```python
from build123d import *

# Parameters (mm, degrees)
SKETCH_1_W          = 15
SKETCH_1_H          = 3
SKETCH_2_R          = 2.1
CUT_EXTRUDE_1_DEPTH = 10


with BuildPart() as part:
    # 草图1 → 旋转1 (revolve)
    with BuildSketch(Plane.XY, mode=Mode.PRIVATE) as revolve_1_sk:
        with Locations((83.58, 1.5)):
            Rectangle(SKETCH_1_W, SKETCH_1_H)
    revolve(revolve_1_sk.sketch.rotate(Axis((0, 0, 0), (0, 1, 0)), 90), axis=Axis((0, 0, 0), (0, 1, 0)))

    # 草图2 → 切除-拉伸1 (cut)
    with BuildSketch(Plane(origin=(0, 3, 0), x_dir=(1, 0, 0), z_dir=(0, 1, 0))):
        with Locations(Location((-83.9, 0, 0), (0, 0, 270))):
            Circle(SKETCH_2_R)
        with Locations(Location((-59.326258942, 59.326258942, 0), (0, 0, 270))):
            Circle(SKETCH_2_R)
        with Locations(Location((0, 83.9, 0), (0, 0, 270))):
            Circle(SKETCH_2_R)
        with Locations(Location((59.326258942, 59.326258942, 0), (0, 0, 270))):
            Circle(SKETCH_2_R)
        with Locations(Location((83.9, 0, 0), (0, 0, 270))):
            Circle(SKETCH_2_R)
        with Locations(Location((59.326258942, -59.326258942, 0), (0, 0, 270))):
            Circle(SKETCH_2_R)
        with Locations(Location((0, -83.9, 0), (0, 0, 270))):
            Circle(SKETCH_2_R)
        with Locations(Location((-59.326258942, -59.326258942, 0), (0, 0, 270))):
            Circle(SKETCH_2_R)
    extrude(amount=-CUT_EXTRUDE_1_DEPTH, mode=Mode.SUBTRACT)


solid = part.part
```
Geometry check sheet. Reference: the model listing, model coordinates, mm. Give positions to 0.01 mm unless a question says otherwise; leave off trailing zeros. Order: outer loops, then holes, each group sorted by start corner. A loop starts at its lowest first (then second) coordinate and runs counter-clockwise, first axis right, second up. Notation, with made-up numbers: (48, 61.25) - (95, 61.25) arc R12 ccw to (95, 66.25) - close; hole circle Ø2 at (67, 41). An arc over 180 degrees is marked (long way). Answer in a Markdown table with one row per item. Add a question column.
Q1. Mould release check, pull along Z, two halves, no side actions. Record for faces 1 (the cylindrical face through (-27.358, 1.521, -86.874)), 2 (the flat face through (-54, 0, 54)), 3 (the cylindrical face through (-60.604, 1.521, -60.993)): pulls with the +Z half, pulls with the -Z half, needs draft (parallel to the pull), parting line crosses it, or undercut.
Q2. Material ranges on probe 1 along X at (y, z) = (1, 0); probe 2 along Z at (x, y) = (-1.5, 2.55); probe 3 along X at (y, z) = (0.3, -1), recorded low to high. Write a range as from..to.
Q3. Cross-section at B-B, the plane z = -63.5. Enter the section's corners in (x, y).
Q4. Cross-section at A-A, the plane x = 52. Enter the section's corners in (y, z), then the cut area to 3 significant figures.
Q5. Cross-section at C-C, the plane y = 0.9. Count the separate pieces of the cut face and the enclosed holes in it, then the cut area to 3 significant figures.
Q6. Gauge pin test, flat end, axial feed: pin 1 (2.5 mm diameter, centred on x = 0, z = -83.9, fed in from +Y). Record the tip position at first contact, or that the pin passes through.
Check values:
| question | item | result |
|---|---|---|
| 1 | face 1 | parting line crosses it |
| 1 | face 2 | needs draft |
| 1 | face 3 | undercut |
| 2 | probe 1 | x = -91.08..-86, -81.8..-76.08, 76.08..81.8, 86..91.08 |
| 2 | probe 2 | z = -91.07..-85.37, -82.43..-76.07, 76.07..82.43, 85.37..91.07 |
| 2 | probe 3 | x = -91.07..-85.75, -82.05..-76.07, 76.07..82.05, 85.75..91.07 |
| 3 | outline | (-65.29, 0) - (-41.9, 0) - (-41.9, 3) - (-65.29, 3) - close; (41.9, 0) - (65.29, 0) - (65.29, 3) - (41.9, 3) - close |
| 4 | outline | (0, -74.78) - (3, -74.78) - (3, -55.54) - (0, -55.54) - close; (0, 55.54) - (3, 55.54) - (3, 74.78) - (0, 74.78) - close |
| 4 | area | 115 mm^2 |
| 5 | separate pieces | 1 |
| 5 | enclosed holes | 9 |
| 5 | area | 7,770 mm^2 |
| 6 | pin 1 | passes through |
